Geometry: see drawing. Coordinates: mm, zero at the bounding-box minimum. Round coordinates to 2 decimals unless told otherwise and drop trailing zeros. Order: outer loops, then holes, each group sorted by start corner. A loop starts at its lowest first (then second) coordinate and runs counter-clockwise, first axis right, second up. Notation, with made-up numbers: M 85.25,-11 L 143.25,-11 A20 cw 143.25,21 Z; hole C -37.5,-24 d7. An arc over 180 degrees is marked long. Answer in a Markdown table with one row per item. Add a question column.
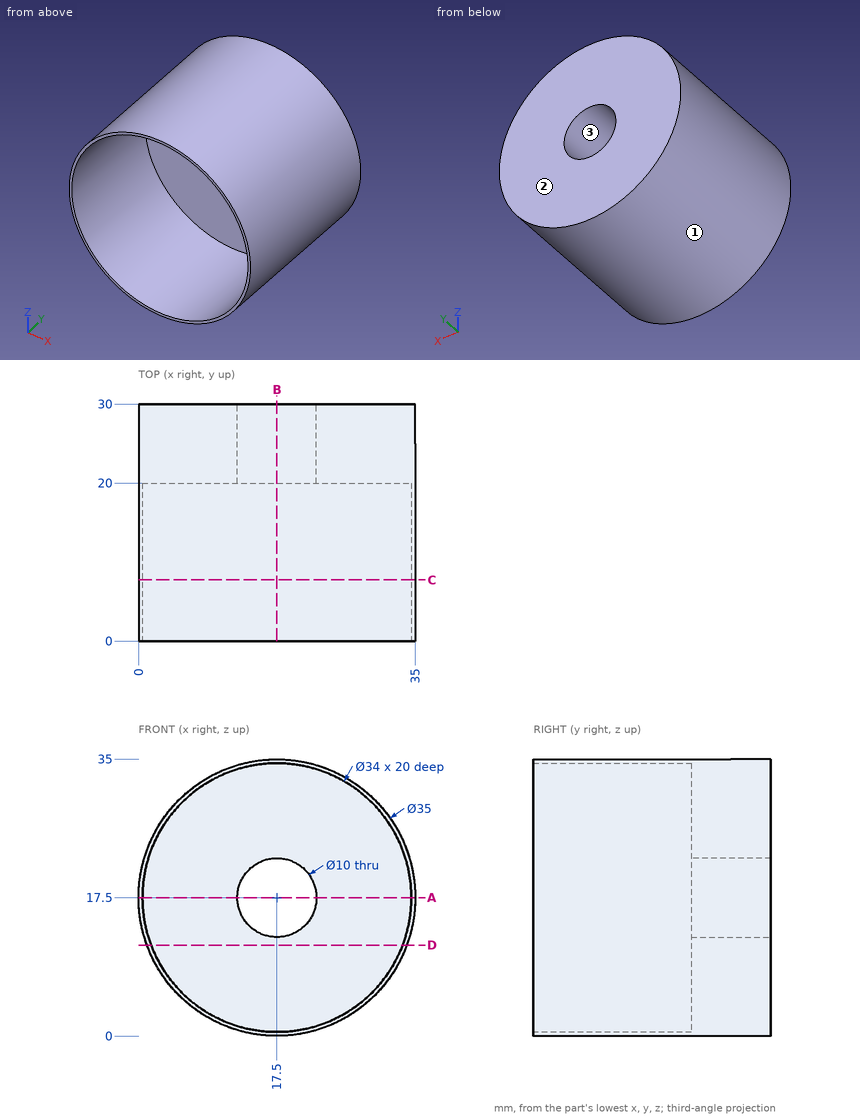
(1) Line query: line 1 (Z direction, x = 17.5, y = 10.5); line 2 (Y direction, x = 24, z = 20.5). Output: solid intervals per line, ascending. Write a range as from..to.
(2) Cut plane C-C (y = 7.75). Return loops of the section in (x, z), and give its area (3 significant figures).
(3) Cut plane B-B (x = 17.5). Return loops of the section in (y, z), and give its area (3 significant figures).
(4) Cut plane A-A (z = 17.5). Return loops of the section in (x, y), and give its area (3 significant figures).
(5) Cut plane D-D (z = 11.5). Return loops of the section in (x, y).
(6) Pin query (flat end, axial travel): pin 1 (1 mm diameter, centred on y = 17, z = 6.5, fed in from -X); pin 2 (2 mm diameter, centred on y = 24.5, z = 3.5, fed in from +X); pin 3 (2 mm diameter, centred on x = 11, z = 26.5, fed in from -Y). Return the tip coordinate at first contact, or that it passes through.
(7) Draft query along X for the marked faces 1, 2 and 3. Return one class per face: +X half, -X half, draft (parallel to the pull), parting line (faces both ways), or undercut.
Answer list:
| question | item | result |
|---|---|---|
| 1 | line 1 | 0..0.5, 34.5..35 |
| 1 | line 2 | 20..30 |
| 2 | outline | C 17.5,17.5 d35; hole C 17.5,17.5 d34 |
| 2 | area | 54.2 mm² |
| 3 | outline | M 0,0 L 30,0 L 30,12.5 L 20,12.5 L 20,0.5 L 0,0.5 Z; M 0,34.5 L 20,34.5 L 20,22.5 L 30,22.5 L 30,35 L 0,35 Z |
| 3 | area | 270 mm² |
| 4 | outline | M 0,0 L 0.5,0 L 0.5,20 L 12.5,20 L 12.5,30 L 0,30 Z; M 22.5,20 L 34.5,20 L 34.5,0 L 35,0 L 35,30 L 22.5,30 Z |
| 4 | area | 270 mm² |
| 5 | outline | M 1.06,0 L 1.59,0 L 1.59,20 L 33.41,20 L 33.41,0 L 33.94,0 L 33.94,30 L 1.06,30 Z |
| 6 | pin 1 | x = 3.5 |
| 6 | pin 2 | x = 29.22 |
| 6 | pin 3 | y = 20 |
| 7 | face 1 | parting line |
| 7 | face 2 | draft |
| 7 | face 3 | undercut |
